Verification items for the finished model (mm, model axes). Face numbers are marked on the shaded views. A direction names the side the tool comes from. Round coordinates to 2 decimals unless told otherwise and drop trailing zeros. Order: outer loops, then holes, each group sorted by start corner. A loop starts at its lowest first (then second) coordinate and runs counter-clockwise, first axis right, second up. Notation, with made-up numbers: M 12.5,-35 L 31.5,-35 A20 cw 31.5,-13 Z; hole C 42.5,33 d6. An arc over 180 degrees is marked long. Return JSON: item names as keys, results as strings. Group by question number.
from build123d import *

# Parameters (mm, degrees)
AUFSATZ_LINEAR_AUSTRAGEN1_DEPTH = 60
SKIZZE2_R                       = 20
SKIZZE2_R_2                     = 3
SCHNITT_LINEAR_AUSTRAGEN1_DEPTH = 20
SKIZZE3_R                       = 3
SCHNITT_LINEAR_AUSTRAGEN2_DEPTH = 20
SKIZZE4_R                       = 7
SCHNITT_LINEAR_AUSTRAGEN3_DEPTH = 10
SKIZZE5_R                       = 3
SCHNITT_LINEAR_AUSTRAGEN4_DEPTH = 10


with BuildPart() as part:
    # Skizze1 → Aufsatz-Linear austragen1 (new, symmetric)
    with BuildSketch(Plane.XY):
        Polygon((-70, 0), (0, 0), (0, -60), (-4, -60), (-4, -4), (-70, -4), align=None)
    extrude(amount=AUFSATZ_LINEAR_AUSTRAGEN1_DEPTH, both=True)

    # Skizze2 → Schnitt-Linear austragen1 (cut)
    with BuildSketch(Plane(origin=(0, 0, 0), x_dir=(1, 0, 0), z_dir=(0, 1, 0))):
        with Locations(Location((-41, 0, 0), (0, 0, 270))):
            Circle(SKIZZE2_R)
        with Locations(Location((-17.5, 23.5, 0), (0, 0, 270))):
            Circle(SKIZZE2_R_2)
        with Locations(Location((-64.5, 23.5, 0), (0, 0, 180))):
            Circle(SKIZZE2_R_2)
        with Locations(Location((-17.5, -23.5, 0), (0, 0, 180))):
            Circle(SKIZZE2_R_2)
        with Locations(Location((-64.5, -23.5, 0), (0, 0, 270))):
            Circle(SKIZZE2_R_2)
    extrude(amount=-SCHNITT_LINEAR_AUSTRAGEN1_DEPTH, mode=Mode.SUBTRACT)

    # Skizze3 → Schnitt-Linear austragen2 (cut)
    with BuildSketch(Plane(origin=(0, 0, 0), x_dir=(0, 0, -1), z_dir=(1, 0, 0))):
        with Locations(Location((40, -42, 0), (0, 0, 90))):
            Circle(SKIZZE3_R)
        with Locations((-40, -42)):
            Circle(SKIZZE3_R)
        with Locations(Location((20, -42, 0), (0, 0, 90))):
            Circle(SKIZZE3_R)
        with Locations((-20, -42)):
            Circle(SKIZZE3_R)
    extrude(amount=-SCHNITT_LINEAR_AUSTRAGEN2_DEPTH, mode=Mode.SUBTRACT)

    # Skizze4 → Schnitt-Linear austragen3 (cut)
    with BuildSketch(Plane(origin=(0, 0, 0), x_dir=(0, 0, -1), z_dir=(1, 0, 0))):
        with Locations((23, -62)):
            Circle(SKIZZE4_R)
        with Locations((-23, -62)):
            Circle(SKIZZE4_R)
    extrude(amount=-SCHNITT_LINEAR_AUSTRAGEN3_DEPTH, mode=Mode.SUBTRACT)

    # Skizze5 → Schnitt-Linear austragen4 (cut)
    with BuildSketch(Plane(origin=(0, 0, 0), x_dir=(1, 0, 0), z_dir=(0, 1, 0))):
        with Locations(Location((-58, -52, 0), (0, 0, 270))):
            Circle(SKIZZE5_R)
        with Locations(Location((-35, -52, 0), (0, 0, 270))):
            Circle(SKIZZE5_R)
        with Locations(Location((-12, -52, 0), (0, 0, 270))):
            Circle(SKIZZE5_R)
        with Locations(Location((-58, 52, 0), (0, 0, 180))):
            Circle(SKIZZE5_R)
        with Locations(Location((-35, 52, 0), (0, 0, 180))):
            Circle(SKIZZE5_R)
        with Locations(Location((-12, 52, 0), (0, 0, 180))):
            Circle(SKIZZE5_R)
    extrude(amount=-SCHNITT_LINEAR_AUSTRAGEN4_DEPTH, mode=Mode.SUBTRACT)


solid = part.part
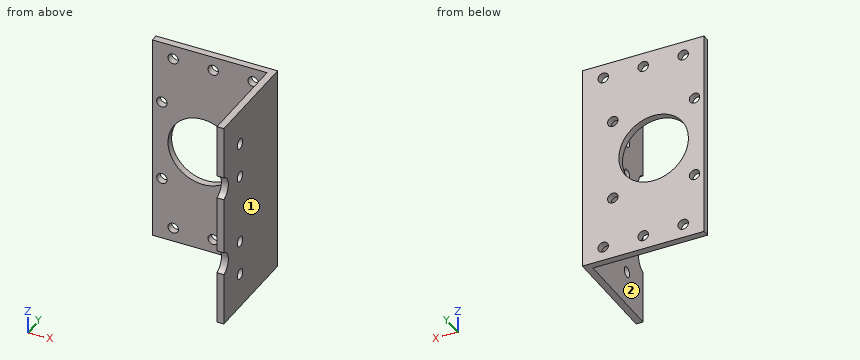
1. Cross-section at B-B (y = -42). Enter the section's corners in (x, z).
2. Go/stop test with flat-tipped pins: pin 1 (6 mm diameter, centred on y = -45.5, z = -23, fed in from -X); pin 2 (12 mm diameter, centred on x = -52.5, z = -29.5, fed in from -Y). Record where each tip stops, or that it passes through.
3. Cross-section at A-A (z = 0). Enter the section's corners in (x, y).
4. Thickness scan on line 1 along X through (y, z) = (-1, 52); line 2 along Y through (x, z) = (-14, -15). Record the ranges inside material, lowest first. Write a range as from..to.
5. Cross-section at C-C (x = -48.5). Enter the section's corners in (y, z), plus the area to 3 significant figures.
6. Access from +Z, -Z, +X, -X, +Y, -Y to the whole of each face (thin tool, end or side, straight path). Record for the marked faces 1 and 2.
7. Cross-section at D-D (z = 52). Enter the section's corners in (x, y).
Computed:
{
 "1": {"outline": "M -4,-60 L 0,-60 L 0,-43 L -4,-43 Z; M -4,-37 L 0,-37 L 0,-23 L -4,-23 Z; M -4,-17 L 0,-17 L 0,17 L -4,17 Z; M -4,23 L 0,23 L 0,37 L -4,37 Z; M -4,43 L 0,43 L 0,60 L -4,60 Z"},
 "2": {"pin 1": "stops at x = -4", "pin 2": "stops at y = -4"},
 "3": {"outline": "M -70,-4 L -61,-4 L -61,0 L -70,0 Z; M -21,-4 L -4,-4 L -4,-60 L 0,-60 L 0,0 L -21,0 Z"},
 "4": {"line 1": "x = -70..-61, -55..-38, -32..-15, -9..0", "line 2": "y = -4..0"},
 "5": {"outline": "M -4,-60 L 0,-60 L 0,-18.54 L -4,-18.54 Z; M -4,18.54 L 0,18.54 L 0,60 L -4,60 Z", "area": "332 mm²"},
 "6": {"face 1": "+Z, -Z, +X, +Y, -Y", "face 2": "+Z, -Z, -X, -Y"},
 "7": {"outline": "M -70,-4 L -61,-4 L -61,0 L -70,0 Z; M -55,-4 L -38,-4 L -38,0 L -55,0 Z; M -32,-4 L -15,-4 L -15,0 L -32,0 Z; M -9,-4 L -4,-4 L -4,-60 L 0,-60 L 0,0 L -9,0 Z"}
}
